```python
from build123d import *

# Parameters (mm, degrees)
SKETCH1_W           = 46
SKETCH1_H           = 40
BOSS_EXTRUDE1_DEPTH = 3
SKETCH3_W           = 35
SKETCH3_H           = 30
CUT_EXTRUDE1_DEPTH  = 3
SKETCH4_W           = 5
SKETCH4_H           = 3
CUT_EXTRUDE3_DEPTH  = 3
SKETCH6_W           = 7
SKETCH6_H           = 3
BOSS_EXTRUDE2_DEPTH = 5
SKETCH7_W           = 11
SKETCH7_H           = 40
CUT_EXTRUDE4_DEPTH  = 3
SKETCH8_W           = 5
SKETCH8_H           = 3
BOSS_EXTRUDE3_DEPTH = 30
SKETCH9_W           = 5
SKETCH9_H           = 3
SKETCH9_W_2         = 10
BOSS_EXTRUDE4_DEPTH = 3
FILLET2_R           = 4


with BuildPart() as part:
    # Sketch1 → Boss-Extrude1 (new body)
    with BuildSketch(Plane(origin=(0, 0, 0), x_dir=(1, 0, 0), z_dir=(0, 1, 0))):
        Rectangle(SKETCH1_W, SKETCH1_H)
    extrude(amount=BOSS_EXTRUDE1_DEPTH)

    # Sketch3 → Cut-Extrude1 (cut)
    with BuildSketch(Plane(origin=(0, 3, 0), x_dir=(1, 0, 0), z_dir=(0, 1, 0))):
        with Locations((5.5, 5)):
            Rectangle(SKETCH3_W, SKETCH3_H)
    extrude(amount=-CUT_EXTRUDE1_DEPTH, mode=Mode.SUBTRACT)

    # Sketch4 → Cut-Extrude3 (cut)
    with BuildSketch(Plane(origin=(0, 0, 10), x_dir=(-1, 0, 0), z_dir=(0, 0, -1))):
        with Locations((-15.5, 1.5)):
            Rectangle(SKETCH4_W, SKETCH4_H)
        with Locations((-5.5, 1.5)):
            Rectangle(SKETCH4_W, SKETCH4_H)
        with Locations((4.5, 1.5)):
            Rectangle(SKETCH4_W, SKETCH4_H)
    extrude(amount=-CUT_EXTRUDE3_DEPTH, mode=Mode.SUBTRACT)

    # Sketch6 → Boss-Extrude2 (add)
    with BuildSketch(Plane(origin=(23, 0, 0), x_dir=(0, 0, -1), z_dir=(1, 0, 0))):
        with Locations((-16.5, 1.5)):
            Rectangle(SKETCH6_W, SKETCH6_H)
    extrude(amount=BOSS_EXTRUDE2_DEPTH)

    # Sketch7 → Cut-Extrude4 (cut)
    with BuildSketch(Plane.XZ):
        with Locations((-17.5, 0)):
            Rectangle(SKETCH7_W, SKETCH7_H)
    extrude(amount=-CUT_EXTRUDE4_DEPTH, mode=Mode.SUBTRACT)

    # Sketch8 → Boss-Extrude3 (add)
    with BuildSketch(Plane(origin=(0, 0, 10), x_dir=(-1, 0, 0), z_dir=(0, 0, -1))):
        with Locations((9.5, 1.5)):
            Rectangle(SKETCH8_W, SKETCH8_H)
    extrude(amount=BOSS_EXTRUDE3_DEPTH)

    # Sketch9 → Boss-Extrude4 (add)
    with BuildSketch(Plane.ZY.offset(12)):
        with Locations((-17.5, 1.5)):
            Rectangle(SKETCH9_W, SKETCH9_H)
        with Locations((-7.5, 1.5)):
            Rectangle(SKETCH9_W, SKETCH9_H)
        with Locations((2.5, 1.5)):
            Rectangle(SKETCH9_W, SKETCH9_H)
        with Locations((15, 1.5)):
            Rectangle(SKETCH9_W_2, SKETCH9_H)
    extrude(amount=BOSS_EXTRUDE4_DEPTH)

    # Fillet2
    fillet2_edges = [part.edges().sort_by_distance(p)[0] for p in [
        (-7, 1.5, -20),
        (-15, 1.5, 20),
        (28, 1.5, 20),
    ]]
    fillet(fillet2_edges, radius=FILLET2_R)


solid = part.part
```
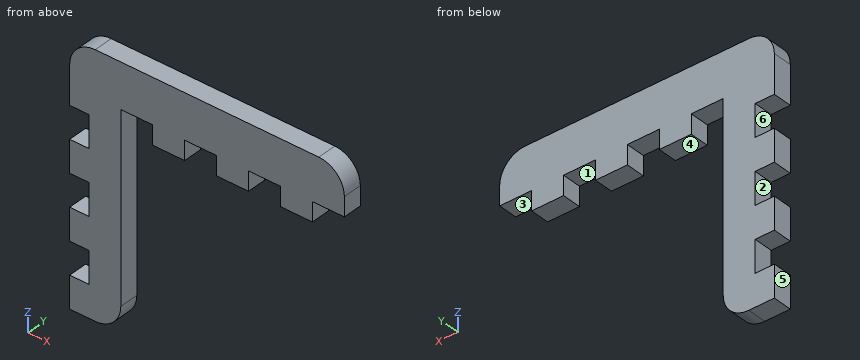
Build history of the part. All positions in model axes, mm. Face numbers are marked on the shaded views. A direction names the side the tool comes from. Give positions to 0.01 mm unless a question says otherwise; leave off trailing zeros. Loops run counter-clockwise (first coordinate to the right, second up) from the corner with the lowest first, then second, coordinate; pieces in that order, holes last.
Item 1: Which spindle directions (+Z, -Z, +X, -X, +Y, -Y) get a long thin tool onto all of the face, cutting with end or side? Do the marked faces 1, 2 and 3. Say none if no direction does.
Answers follow:
face 1: -Z, +Y, -Y
face 2: -X, +Y, -Y
face 3: -Z, +X, +Y, -Y
Item 2: Slice it at A-A, the plane z = 12. List the corners of the cut face in (x, y).
Answers follow:
outline: (-15, 0) - (-7, 0) - (-7, 3) - (-15, 3) - close; (-2, 0) - (3, 0) - (3, 3) - (-2, 3) - close; (8, 0) - (13, 0) - (13, 3) - (8, 3) - close; (18, 0) - (23, 0) - (23, 3) - (18, 3) - close
Item 3: Pull direction Z, two halves, no side cores. Call the marked faces 4, 5 and 6: released by +Z, released by -Z, zero draft, split by the parting line, or undercut.
Answers follow:
face 4: released by -Z
face 5: zero draft
face 6: undercut
Item 4: Slice it at D-D, the plane z = 1. List the corners of the cut face in (x, y), and give its area (3 significant figures).
Answers follow:
outline: (-15, 0) - (-7, 0) - (-7, 3) - (-15, 3) - close
area: 24.0 mm2
Item 5: Drill centre lines: line 1 (X direction, y = 2.5, z = 11.5); line 2 (Z direction, x = -13, y = 2.5); line 3 (Z direction, x = 15.5, y = 2.55). Where is each one in solid material? Low to high.
Answers follow:
line 1: x = -15 to -7, -2 to 3, 8 to 13, 18 to 23
line 2: z = -20 to -15, -10 to -5, 0 to 5, 10 to 19.46
line 3: z = 13 to 20
Item 6: Flat gauge pins, fed straight in: pin 1 (1.5 mm diameter, centred on x = 9.5, y = 1, fed in from -Z); pin 2 (1 mm diameter, centred on y = 2.5, z = -12, fed in from -X); pin 3 (1.5 mm diameter, centred on x = -13.5, y = 1.5, fed in from +Z). Where does each tip first touch, or does it go through?
Answers follow:
pin 1: stops at z = 10
pin 2: stops at x = -12
pin 3: stops at z = 19.6
Item 7: Slice it at C-C, the plane x = 7.5. List the corners of the cut face in (y, z).
Answers follow:
outline: (0, 13) - (3, 13) - (3, 20) - (0, 20) - close
